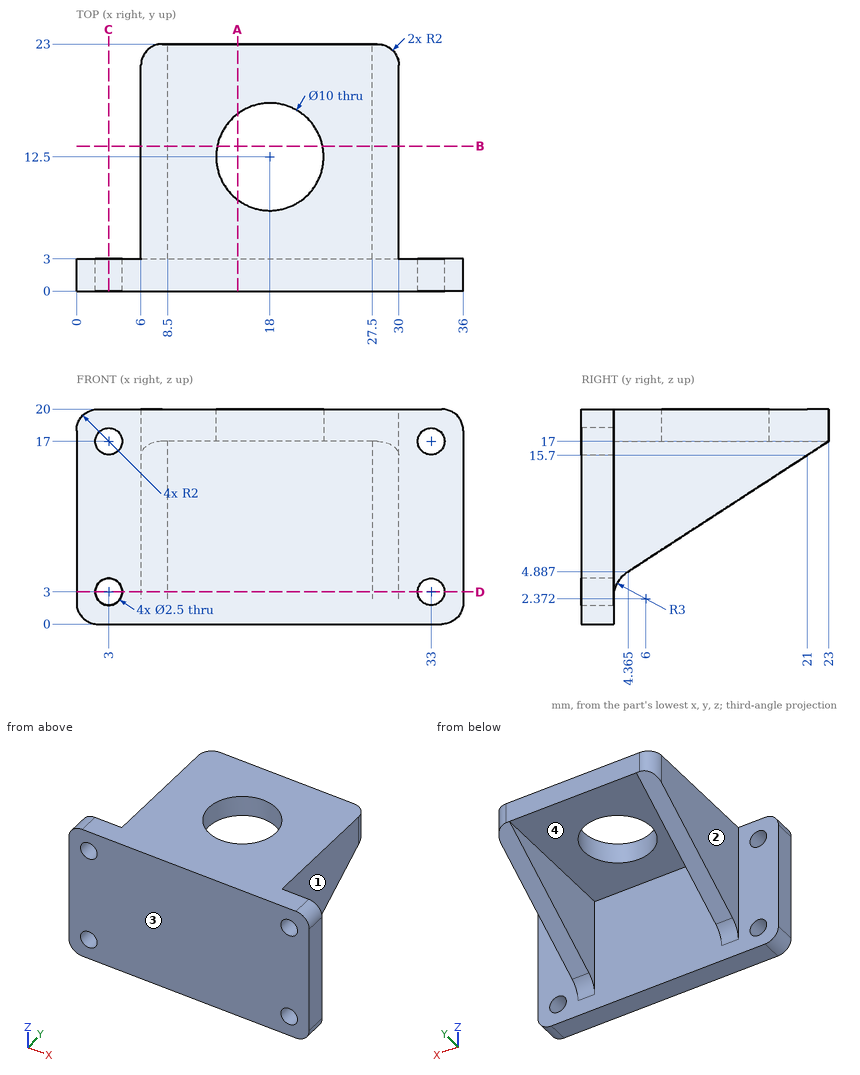
Geometry: see drawing. Coordinates: mm, zero at the bounding-box minimum. A direction names the side the tool comes from. Round coordinates to 2 decimals unless told otherwise and drop trailing zeros. Write each loop counter-clockwise with the first axis right and the second up, starting at its lowest first coordinate (ties: lowest second). Pieces come first, ordered by that corner, then holes.
Item 1: Section query A-A (x = 15). Return loops of the section in (y, z), plus the area to 3 significant figures.
Item 2: Set-up query: the marked faces 1, 2, 3 and 4. Return all of +Z, -Z, +X, -X, +Y, -Y with unobstructed straight access to the full face (end or side cutting, diameter ignored); none if empty.
Item 3: Material intervals for L1, parallel to X at y = 13.75, z = 14.5; L2, parallel to X at y = 1.75, z = 17; L3, parallel to Z at x = 10, y = 9.5, sorted ascending.
Item 4: Section query C-C (x = 3). Return loops of the section in (y, z), plus the area to 3 significant figures.
Item 5: Section query B-B (y = 13.5). Return loops of the section in (x, z) (1 decimal).
Item 6: Pin query (flat end, axial travel): P1, Ø5.5, axis at x = 14, y = 9.5, coming from the -Z side; P2, Ø4.5, axis at y = 15.5, z = 9.5, coming from the +X side; P3, Ø6, axis at x = 23, z = 11, coming from the +Y side. Return the tip coordinate at first contact, or that it passes through.
Item 7: Section query D-D (z = 3). Return loops of the section in (x, y).
Completed:
1. outline: (0, 0) - (3, 0) - (3, 17) - (8.5, 17) - (8.5, 20) - (0, 20) - close; (16.5, 17) - (23, 17) - (23, 20) - (16.5, 20) - close
1. area: 96.0 mm2
2. face 1: +Z, -Z, +X, +Y
2. face 2: +Z, -Z, -X, +Y
2. face 3: +Z, -Z, +X, -X, -Y
2. face 4: -Z, +Y
3. L1: x = 6 to 8.5, 27.5 to 30
3. L2: x = 0 to 1.75, 4.25 to 31.75, 34.25 to 36
3. L3: z = 17 to 20
4. outline: (0, 0) - (3, 0) - (3, 1.75) - (0, 1.75) - close; (0, 4.25) - (3, 4.25) - (3, 15.75) - (0, 15.75) - close; (0, 18.25) - (3, 18.25) - (3, 20) - (0, 20) - close
4. area: 45.0 mm2
5. outline: (6, 10.8) - (8.5, 10.8) - (8.5, 17) - (13.1, 17) - (13.1, 20) - (6, 20) - close; (22.9, 17) - (27.5, 17) - (27.5, 10.8) - (30, 10.8) - (30, 20) - (22.9, 20) - close
6. P1: stops at z = 17
6. P2: stops at x = 30
6. P3: stops at y = 3
7. outline: (0, 0) - (1.75, 0) - (1.75, 3) - (0, 3) - close; (4.25, 0) - (31.75, 0) - (31.75, 3) - (30, 3) - (30, 3.07) - (27.5, 3.07) - (27.5, 3) - (8.5, 3) - (8.5, 3.07) - (6, 3.07) - (6, 3) - (4.25, 3) - close; (34.25, 0) - (36, 0) - (36, 3) - (34.25, 3) - close
